Print and shaded views of the part. All mm, measured from the part's lowest x, y and z. A direction names the side the tool comes from. Round coordinates to 2 decimals unless told otherwise and drop trailing zeros. Loops run counter-clockwise (first coordinate to the right, second up) from the corner with the lowest first, then second, coordinate; pieces in that order, holes last. Notation, with made-up numbers: (84.25, 49.5) - (112.25, 49.5) arc R10 cw to (112.25, 64.5) - close; hole circle Ø2 at (75.5, 11.5). An arc over 180 degrees is marked (long way). Use one line per item in the form item = value.
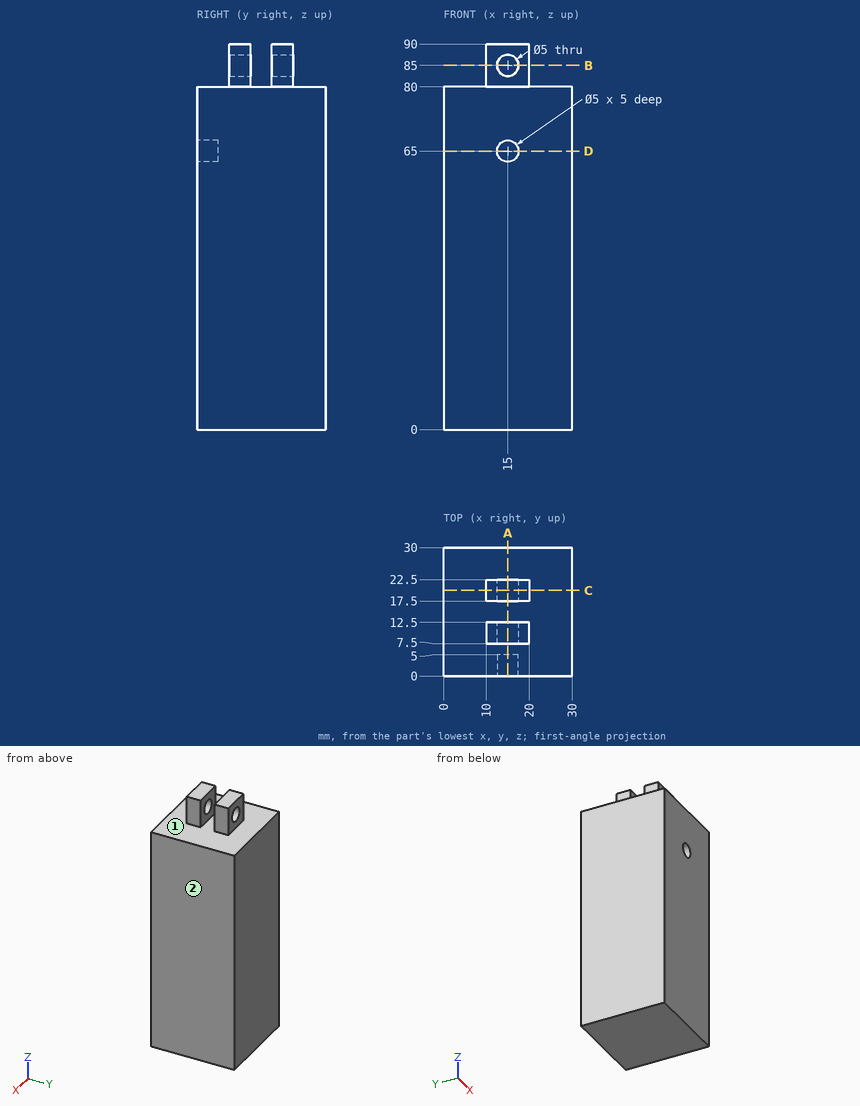
1) Slice it at C-C (y = 20). Write the cut outline in (x, z).
Report:
outline = (0, 0) - (30, 0) - (30, 80) - (20, 80) - (20, 90) - (10, 90) - (10, 80) - (0, 80) - close; hole circle Ø5 at (15, 85)
2) Drill centre lines: probe 1 along Z at (x, y) = (15, 3.3); probe 2 along Z at (x, y) = (15, 21.25); probe 3 along X at (y, z) = (3.4, 65). Where is each one in solid material? Low to high.
Report:
probe_1 = 0 to 62.5, 67.5 to 80
probe_2 = 0 to 82.5, 87.5 to 90
probe_3 = 0 to 12.5, 17.5 to 30
3) Flat gauge pins, fed straight in: pin 1 (8 mm diameter, centred on x = 15.5, z = 84.5, fed in from +Y); pin 2 (1.5 mm diameter, centred on y = 19, z = 83.5, fed in from -X); pin 3 (3 mm diameter, centred on x = 16.5, z = 82.5, fed in from -Y). Where does each tip first touch, or does it go through?
Report:
pin_1 = 22.5
pin_2 = 10
pin_3 = 7.5
4) Slice it at D-D (z = 65). Write the cut outline in (x, y), plus the area to 3 significant figures.
Report:
outline = (0, 0) - (12.5, 0) - (12.5, 5) - (17.5, 5) - (17.5, 0) - (30, 0) - (30, 30) - (0, 30) - close
area = 875 mm^2
5) Slice it at A-A (x = 15). Write the cut outline in (y, z).
Report:
outline = (0, 0) - (30, 0) - (30, 80) - (22.5, 80) - (22.5, 82.5) - (17.5, 82.5) - (17.5, 80) - (12.5, 80) - (12.5, 82.5) - (7.5, 82.5) - (7.5, 80) - (0, 80) - (0, 67.5) - (5, 67.5) - (5, 62.5) - (0, 62.5) - close; (7.5, 87.5) - (12.5, 87.5) - (12.5, 90) - (7.5, 90) - close; (17.5, 87.5) - (22.5, 87.5) - (22.5, 90) - (17.5, 90) - close
6) Tool access for the marked faces 1 and 2: list every direction of +Z, -Z, +X, -X, +Y, -Y with a clear straight run to the whole face (end or side of a thin tool).
Report:
face_1 = +Z
face_2 = +Z, -Z, +X, +Y, -Y
7) Slice it at B-B (z = 85). Write the cut outline in (x, y), plus the area to 3 significant figures.
Report:
outline = (10, 7.5) - (12.5, 7.5) - (12.5, 12.5) - (10, 12.5) - close; (10, 17.5) - (12.5, 17.5) - (12.5, 22.5) - (10, 22.5) - close; (17.5, 7.5) - (20, 7.5) - (20, 12.5) - (17.5, 12.5) - close; (17.5, 17.5) - (20, 17.5) - (20, 22.5) - (17.5, 22.5) - close
area = 50.0 mm^2
